```python
from build123d import *

# Parameters (mm, degrees)
ESQUISSE1_R             = 1.5
BOSS_EXTRU_2_DEPTH      = 40
ESQUISSE3_R             = 1.5
BOSS_EXTRU_3_DEPTH      = 10
BOSS_EXTRU_3_DEPTH_BACK = 30


with BuildPart() as part:
    # Esquisse1 → Boss.-Extru.2 (new body)
    with BuildSketch(Plane.XY):
        Polygon((0, -2.886751346), (2.5, -1.443375673), (2.5, 1.443375673), (0, 2.886751346), (-2.5, 1.443375673), (-2.5, -1.443375673), align=None)
        Circle(ESQUISSE1_R, mode=Mode.SUBTRACT)
    extrude(amount=BOSS_EXTRU_2_DEPTH)

    # Esquisse3 → Boss.-Extru.3 (add, two sides)
    with BuildSketch(Plane(origin=(0, 0, 0), x_dir=(-1, 0, 0), z_dir=(0, 0, -1))) as boss_extru_3_sk:
        Circle(ESQUISSE3_R)
    extrude(amount=BOSS_EXTRU_3_DEPTH)
    extrude(boss_extru_3_sk.sketch, amount=-BOSS_EXTRU_3_DEPTH_BACK)


solid = part.part
```
Geometry check sheet. Reference: the model listing, model coordinates, mm. A direction names the side the tool comes from. Give positions to 0.01 mm unless a question says otherwise; leave off trailing zeros. Write each loop counter-clockwise with the first axis right and the second up, starting at its lowest first coordinate (ties: lowest second). Pieces come first, ordered by that corner, then holes.
1) Section check A-A, the plane z = 31.5. Record the boundary of the cut face in (x, y).
2) Section check B-B, the plane y = 0. Record the boundary of the cut face in (x, z), and give its area (3 significant figures).
3) Access from +Z, -Z, +X, -X, +Y, -Y to the whole of each face (thin tool, end or side, straight path). Record for faces 1 (the flat face through (0, 0, -10)), 2 (the cylindrical face through (1.5, 0.07, -4.93)).
4) Gauge pin test, flat ends, axial feed: pin 1 (2 mm diameter, centred on y = 1.5, z = 9, fed in from -X); pin 2 (2 mm diameter, centred on x = -0.5, z = 15, fed in from +Y). Record the tip position at first contact, or that the pin passes through.
5) Section check D-D, the plane z = -2. Record the boundary of the cut face in (x, y), and give its area (3 significant figures).
6) Section check C-C, the plane z = 4.5. Record the boundary of the cut face in (x, y), and give its area (3 significant figures).
7) Release check for a two-part mould opening along Y. For faces 3 (the flat face through (-1.15, -1.24, 0)), 4 (the cylindrical face through (-1.5, 0.07, 34.93)), 5 (the flat face through (0, 0, 30)), 6 (the flat face through (1.267, 2.155, 19.72)) record: pulls with the +Y half, pulls with the -Y half, needs draft (parallel to the pull), parting line crosses it, or undercut.
8) Material ranges on L1, parallel to Y at x = 0, z = 36.5; L2, parallel to Z at x = 0.3, y = -1.35; L3, parallel to Z at x = -0.1, y = -2.55, recorded low to high.
Computed:
1. outline: (-2.5, -1.44) - (0, -2.89) - (2.5, -1.44) - (2.5, 1.44) - (0, 2.89) - (-2.5, 1.44) - close; hole circle Ø3 at (0, 0)
2. outline: (-2.5, 0) - (-1.5, 0) - (-1.5, -10) - (1.5, -10) - (1.5, 0) - (2.5, 0) - (2.5, 40) - (1.5, 40) - (1.5, 30) - (-1.5, 30) - (-1.5, 40) - (-2.5, 40) - close
2. area: 200 mm2
3. face 1: -Z, +X, -X, +Y, -Y
3. face 2: -Z
4. pin 1: stops at x = -2.5
4. pin 2: stops at y = 2.89
5. outline: circle Ø3 at (0, 0)
5. area: 7.07 mm2
6. outline: (-2.5, -1.44) - (0, -2.89) - (2.5, -1.44) - (2.5, 1.44) - (0, 2.89) - (-2.5, 1.44) - close
6. area: 21.7 mm2
7. face 3: needs draft
7. face 4: undercut
7. face 5: undercut
7. face 6: pulls with the +Y half
8. L1: y = -2.89 to -1.5, 1.5 to 2.89
8. L2: z = -10 to 30
8. L3: z = 0 to 40
